```python
from build123d import *

# Parameters (mm, degrees)
SKETCH3_W            = 10
SKETCH3_H            = 12
SKETCH3_R            = 1.5
BOSS_EXTRUDE2_DEPTH  = 1.5
SKETCH3_5_W          = 20
SKETCH3_5_H          = 1.5
BOSS_EXTRUDE4_DEPTH  = 4
SKETCH3_6_W          = 10
SKETCH3_6_H          = 4
BOSS_EXTRUDE5_DEPTH  = 0.25
BOSS_EXTRUDE7_DEPTH  = 2.5
BOSS_EXTRUDE10_DEPTH = 2
BOSS_EXTRUDE11_DEPTH = 24
FILLET5_R            = 1
FILLET6_R            = 1
BOSS_EXTRUDE12_DEPTH = 2


with BuildPart() as part:
    # Sketch3 → Boss-Extrude2 (new body)
    # profile 1 of 2: a face of its own
    with BuildSketch(Plane(origin=(0, 0, 0), x_dir=(1, 0, 0), z_dir=(0, 1, 0))):
        with Locations((7, 11.5)):
            Rectangle(SKETCH3_W, SKETCH3_H)
        with Locations(Location((4.5, 15, 0), (0, 0, 270))):
            Circle(SKETCH3_R, mode=Mode.SUBTRACT)
    # profile 2 of 2: a face of its own
    with BuildSketch(Plane(origin=(0, 0, 0), x_dir=(1, 0, 0), z_dir=(0, 1, 0))):
        with Locations((17, 11.5)):
            Rectangle(SKETCH3_W, SKETCH3_H)
        with Locations(Location((19.5, 15, 0), (0, 0, 270))):
            Circle(SKETCH3_R, mode=Mode.SUBTRACT)
    extrude(amount=BOSS_EXTRUDE2_DEPTH)

    # Sketch3<6> → Boss-Extrude5 (add)
    with BuildSketch(Plane(origin=(0, 0, 0), x_dir=(1, 0, 0), z_dir=(0, 1, 0))):
        with Locations((17, 3.5)):
            Rectangle(SKETCH3_6_W, SKETCH3_6_H)
        with Locations((7, 3.5)):
            Rectangle(SKETCH3_6_W, SKETCH3_6_H)
    extrude(amount=BOSS_EXTRUDE5_DEPTH)



with BuildPart() as body_2:
    # Sketch3<5> → Boss-Extrude4 (new body)
    with BuildSketch(Plane(origin=(0, 0, 0), x_dir=(1, 0, 0), z_dir=(0, 1, 0))):
        with Locations((12, 0.75)):
            Rectangle(SKETCH3_5_W, SKETCH3_5_H)
    extrude(amount=BOSS_EXTRUDE4_DEPTH)


with BuildPart() as part_1:
    add(part.part)

    add(body_2.part)  # Boss-Extrude7 merges body 2
    # Sketch3<8> → Boss-Extrude7 (add)
    with BuildSketch(Plane(origin=(0, 0, 0), x_dir=(1, 0, 0), z_dir=(0, 1, 0))):
        with BuildLine():
            ThreePointArc((0, 1), (0.292893219, 0.292893219), (1, 0))
            Line((1, 0), (2, 0))
            Line((2, 0), (2, 1.5))
            Line((2, 1.5), (2, 5.5))
            Line((2, 5.5), (2, 17.5))
            Line((2, 17.5), (22, 17.5))
            Line((22, 17.5), (22, 5.5))
            Line((22, 5.5), (22, 1.5))
            Line((22, 1.5), (22, 0))
            Line((22, 0), (23, 0))
            ThreePointArc((23, 0), (23.707106781, 0.292893219), (24, 1))
            Line((24, 1), (24, 18.5))
            ThreePointArc((24, 18.5), (23.707106781, 19.207106781), (23, 19.5))
            Line((23, 19.5), (1, 19.5))
            ThreePointArc((1, 19.5), (0.292893219, 19.207106781), (0, 18.5))
            Line((0, 18.5), (0, 1))
        make_face()
    extrude(amount=BOSS_EXTRUDE7_DEPTH)

    # Sketch9 → Boss-Extrude10 (add)
    with BuildSketch(Plane(origin=(0, 0, 0), x_dir=(0, 0, -1), z_dir=(1, 0, 0))):
        Polygon((0, 2.5), (17.5, 2.5), (17.5, 5.5), (13.5, 5.5), (10, 10), (0, 10), align=None)
    extrude(amount=BOSS_EXTRUDE10_DEPTH)

    # Sketch4 → Boss-Extrude11 (add, through all)
    with BuildSketch(Plane(origin=(24, 0, 0), x_dir=(0, 0, -1), z_dir=(1, 0, 0))):
        Polygon((18.5, 2.5), (19.5, 2.5), (19.5, 5.5), (17.5, 5.5), (17.5, 4.5), (17.5, 2.5), align=None)
    extrude(amount=-BOSS_EXTRUDE11_DEPTH)

    # Fillet5
    fillet5_edges = [part_1.edges().sort_by_distance(p)[0] for p in [
        (24, 4, -19.5),
        (0, 4, -19.5),
    ]]
    fillet(fillet5_edges, radius=FILLET5_R)

    # Fillet6
    fillet6_edges = [part_1.edges().sort_by_distance(p)[0] for p in [
        (0, 6.25, 0),
    ]]
    fillet(fillet6_edges, radius=FILLET6_R)

    # Sketch4<4> → Boss-Extrude12 (add)
    with BuildSketch(Plane(origin=(24, 0, 0), x_dir=(0, 0, -1), z_dir=(1, 0, 0))):
        Polygon((0, 2.5), (17.5, 2.5), (17.5, 4.5), (12.540039711, 4.5), (9.040667866, 9), (0, 9), align=None)
    extrude(amount=-BOSS_EXTRUDE12_DEPTH)


solid = part_1.part
```
CAD build for the part. Positions are in the model's coordinates, mm. A direction names the side the tool comes from. Round coordinates to 2 decimals unless told otherwise and drop trailing zeros. Loops run counter-clockwise (first coordinate to the right, second up) from the corner with the lowest first, then second, coordinate; pieces in that order, holes last. Notation, with made-up numbers: (14.5, 37) - (60.5, 37) arc R23 ccw to (60.5, 62) - close; hole circle Ø7 at (17, -26.5). An arc over 180 degrees is marked (long way). Return JSON: item names as keys, results as strings. Group by question number.
Q1. Band-saw the part on D-D on y = 6.5. Give the cut face in (x, z).
Q2. Band-saw the part on A-A on y = 2. Give the cut face in (x, z), plus the area to 3 significant figures.
Q3. Band-saw the part on C-C on z = -2.5. Give the cut face in (x, y), plus the area to 3 significant figures.
Q4. Band-saw the part on B-B on x = 19.5. Give the cut face in (y, z), plus the area to 3 significant figures.
Q5. Flat gauge pins, fed straight in: pin 1 Ø3.5 at (x, z) = (11, -9.5) entering from +Y; pin 2 Ø6 at (x, y) = (14.5, 8) entering from +Z; pin 3 Ø1.8 at (x, z) = (4.5, -15) entering from -Y; pin 4 Ø3 at (x, z) = (12.5, -17.5) entering from +Y. Where does each tip first touch, or does it go through?
Q6. Two-plate mould, pull along Z, no slides. Class faces 1 (the face through (0.986, 7.719, -11.774)), 2 (the face through (12, 1.5, -12)), 3 (the face through (1, 10, -5)): +Z half, -Z half, draft (parallel to the pull), parting line (faces both ways), or undercut.
Q7. Tool access for faces 4 (the face through (23.014, 6.719, -10.815)), 5 (the face through (10, 5.5, -18)), 6 (the face through (20.51, 0.74, -16.11)), 7 (the face through (12, 2, -1.5)), 8 (the face through (12, 4, -1)): list every direction of +Z, -Z, +X, -X, +Y, -Y with a clear straight run to the whole face (end or side of a thin tool).
Q8. Drill centre lines: line 1 along X through (y, z) = (1, -15); line 2 along Z through (x, y) = (11.5, 3); line 3 along X through (y, z) = (4, -16.75). Where is each one in solid material? Low to high. Write a range as [from, to].
Solutions:
{
 "1": {"outline": "(0, -12.72) - (2, -12.72) - (2, 0) - (1, 0) arc R1 ccw to (0, -1) - close; (22, -10.98) - (24, -10.98) - (24, 0) - (22, 0) - close"},
 "2": {"outline": "(0, -18.5) arc R1 ccw to (1, -19.5) - (23, -19.5) arc R1 ccw to (24, -18.5) - (24, -1) arc R1 ccw to (23, 0) - (1, 0) arc R1 ccw to (0, -1) - close; hole (2, -17.5) - (22, -17.5) - (22, -1.5) - (2, -1.5) - close", "area": "147 mm^2"},
 "3": {"outline": "(0, 0) - (24, 0) - (24, 9) - (22, 9) - (22, 0.25) - (2, 0.25) - (2, 10) - (0, 10) - close", "area": "43.0 mm^2"},
 "4": {"outline": "(0, -19.5) - (5.5, -19.5) - (5.5, -17.5) - (1.5, -17.5) - (1.5, -16.5) - (0, -16.5) - close; (0, -13.5) - (1.5, -13.5) - (1.5, -5.5) - (0.25, -5.5) - (0.25, -1.5) - (4, -1.5) - (4, 0) - (0, 0) - close", "area": "31.5 mm^2"},
 "5": {"pin 1": "stops at y = 1.5", "pin 2": "stops at z = -17.5", "pin 3": "passes through", "pin 4": "stops at y = 5.5"},
 "6": {"face 1": "-Z half", "face 2": "undercut", "face 3": "draft"},
 "7": {"face 4": "+X, +Y", "face 5": "-Z, +X, -X, +Y", "face 6": "+Y, -Y", "face 7": "+Y", "face 8": "+Z, +Y"},
 "8": {"line 1": "x = [0, 3], [6, 18], [21, 24]", "line 2": "z = [-19.5, -17.5], [-1.5, 0]", "line 3": "x = [0, 2], [22, 24]"}
}
